Build history of the part. All positions in model axes, mm. A direction names the side the tool comes from. Round coordinates to 2 decimals unless told otherwise and drop trailing zeros. Order: outer loops, then holes, each group sorted by start corner. A loop starts at its lowest first (then second) coordinate and runs counter-clockwise, first axis right, second up. Notation, with made-up numbers: (62, 2) -> (71, 2) arc R21 cw to (71, 35) -> close; hole circle Ø7 at (39.5, 40). An arc over 180 degrees is marked (long way). Answer as a JSON object with one key per item and string values.
from build123d import *

# Parameters (mm, degrees)
BASEHEAD_DEPTH = 7.68
SKETCH3_R      = 6
BASEBODY_DEPTH = 60
CHAMFER1_SIZE  = 0.947


with BuildPart() as part:
    # Sketch-BaseHead → BaseHead (new body)
    with BuildSketch(Plane(origin=(0, 0, 0), x_dir=(0, 0, -1), z_dir=(1, 0, 0))):
        Polygon((10.236420273, 0), (5.118210136, 8.865), (-5.118210136, 8.865), (-10.236420273, 0), (-5.118210136, -8.865), (5.118210136, -8.865), align=None)
    extrude(amount=BASEHEAD_DEPTH)

    # Sketch4 → HeadChamfer (revolve, cut)
    with BuildSketch(Plane(origin=(-0.264637255, 0, 5.916896391), x_dir=(0, 0, -1), z_dir=(0, 1, 0))):
        Polygon((16.153316664, -0.264637255), (14.781896391, -0.264637255), (16.153316664, -0.763793413), align=None)
    revolve(axis=Axis((-4.001564945, 0, 0), (1, 0, 0)), mode=Mode.SUBTRACT)

    # Sketch1 → Revolve1 (revolve)
    with BuildSketch(Plane.XY, mode=Mode.PRIVATE) as revolve1_sk:
        Polygon((7.68, 0), (8.18, 0), (8.18, -8.315), (7.68, -8.865), align=None)
    revolve(revolve1_sk.sketch.rotate(Axis((-4.001564945, 0, 0), (1, 0, 0)), 270), axis=Axis((-4.001564945, 0, 0), (1, 0, 0)))

    # Sketch3 → BaseBody (add)
    with BuildSketch(Plane(origin=(8.18, 0, 0), x_dir=(0, 0, -1), z_dir=(1, 0, 0))):
        Circle(SKETCH3_R)
    extrude(amount=BASEBODY_DEPTH)

    # Chamfer1
    chamfer1_edges = [part.edges().sort_by_distance(p)[0] for p in [
        (68.18, 0, 6),
    ]]
    chamfer(chamfer1_edges, length=CHAMFER1_SIZE)


solid = part.part
1) Probe L1, parallel to X at y = 4, z = 6; L2, parallel to Z at x = 63.5, y = -2.75; L3, parallel to Z at x = 56, y = -1. List the from-to ranges inside material, lowest first. Write a range as from..to.
Checked values:
{"L1": "x = 0..8.18", "L2": "z = -5.33..5.33", "L3": "z = -5.92..5.92"}
2) Flat gauge pins, fed straight in: pin 1 Ø5 at (x, y) = (36, -6.5) entering from -Z; pin 2 Ø3.5 at (y, z) = (6, 3.5) entering from +X; pin 3 Ø2 at (y, z) = (-6, -3.5) entering from +X. Where does each tip first touch, or does it go through?
Checked values:
{"pin 1": "stops at z = -4.47", "pin 2": "stops at x = 68.04", "pin 3": "stops at x = 67.29"}
3) Which spindle directions (+Z, -Z, +X, -X, +Y, -Y) get a long thin tool onto all of the face, cutting with end or side? Do faces 1 (the face through (7.68, 8, 4.4)), 2 (the face through (7.68, 0, -9.2)), 3 (the face through (7.68, -8, 4.4)), 4 (the face through (7.68, -8, -5)), 5 (the face through (37, 0, 6)). Say none if no direction does.
Checked values:
{"face 1": "+Z, +X, +Y", "face 2": "-Z, +X", "face 3": "+Z, +X, -Y", "face 4": "-Z, +X, -Y", "face 5": "+X"}
4) Cut at A-A, the plane x = 28. Give the cut face in (y, z), plus the area to 3 significant figures.
Checked values:
{"outline": "circle Ø12 at (0, 0)", "area": "113 mm²"}
